Drawing for the job (mm, zero at the part's lowest x, y, z). A direction names the side the tool comes from. Give positions to 0.01 mm unless a question says otherwise; leave off trailing zeros. Loops run counter-clockwise (first coordinate to the right, second up) from the corner with the lowest first, then second, coordinate; pieces in that order, holes last. Notation, with made-up numbers: (12, 21.25) -> (40, 21.25) arc R15 cw to (40, 28.25) -> close; hole circle Ø1 at (60, 36). An arc over 180 degrees is marked (long way). Write item = value, one per line.
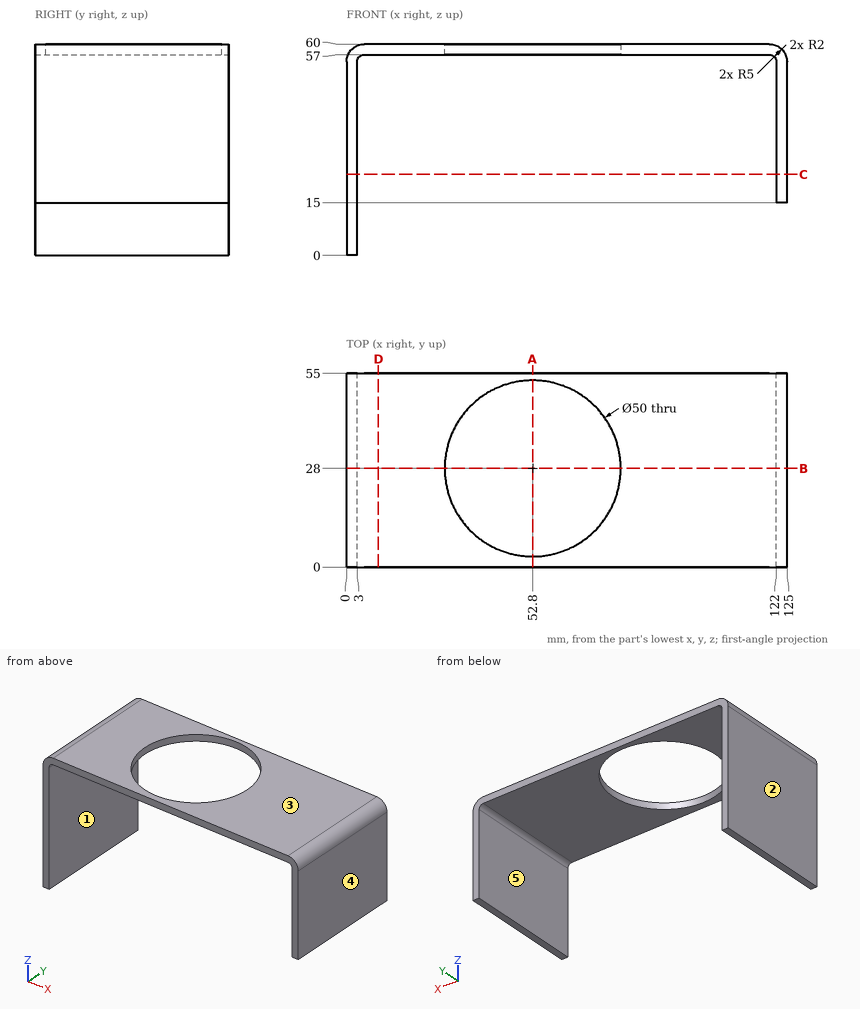
1) Slice it at C-C, the plane z = 23. List the corners of the cut face in (x, y).
Resolved:
outline = (0, 0) -> (3, 0) -> (3, 55) -> (0, 55) -> close; (122, 0) -> (125, 0) -> (125, 55) -> (122, 55) -> close
2) Which spindle directions (+Z, -Z, +X, -X, +Y, -Y) get a long thin tool onto all of the face, cutting with end or side? Do the marked faces 4 and 5. Say none if no direction does.
Resolved:
face_4 = +Z, -Z, +X, +Y, -Y
face_5 = -Z, +Y, -Y
3) Slice it at D-D, the plane x = 9. List the corners of the cut face in (y, z), and give its area (3 significant figures).
Resolved:
outline = (0, 57) -> (55, 57) -> (55, 60) -> (0, 60) -> close
area = 165 mm²
4) Slice it at B-B, the plane y = 28. List the corners of the cut face in (x, z), and give its area (3 significant figures).
Resolved:
outline = (0, 0) -> (3, 0) -> (3, 55) arc R2 cw to (5, 57) -> (27.8, 57) -> (27.8, 60) -> (5, 60) arc R5 ccw to (0, 55) -> close; (77.8, 57) -> (120, 57) arc R2 cw to (122, 55) -> (122, 15) -> (125, 15) -> (125, 55) arc R5 ccw to (120, 60) -> (77.8, 60) -> close
area = 513 mm²
5) Drill centre lines: line 1 along Y through (x, z) = (52, 58); line 2 along X through (y, z) = (13.5, 34); line 3 along Z through (x, y) = (89.5, 52). Where is each one in solid material? Low to high. Write a range as [from, to].
Resolved:
line_1 = [0, 3.01], [52.99, 55]
line_2 = [0, 3], [122, 125]
line_3 = [57, 60]
6) Pull direction X, two halves, no side cores. Call the marked faces 1, 2 and 3: pulls with the +X half, pulls with the -X half, needs draft (parallel to the pull), parting line crosses it, or undercut.
Resolved:
face_1 = undercut
face_2 = pulls with the -X half
face_3 = needs draft
7) Slice it at A-A, the plane x = 52.8. List the corners of the cut face in (y, z), and give its area (3 significant figures).
Resolved:
outline = (0, 57) -> (3, 57) -> (3, 60) -> (0, 60) -> close; (53, 57) -> (55, 57) -> (55, 60) -> (53, 60) -> close
area = 15.0 mm²
8) Drop flat-ended pins along their axis: P1, Ø5, axis at y = 8.5, z = 36, coming from the -X side; P2, Ø3.5, axis at x = 123.5, y = 35.5, coming from the -Z side. Give the stop position or say it passes through.
Resolved:
P1 = 0
P2 = 15
